CAD build for the part. Positions are in the model's coordinates, mm. A direction names the side the tool comes from. Round coordinates to 2 decimals unless told otherwise and drop trailing zeros. Loops run counter-clockwise (first coordinate to the right, second up) from the corner with the lowest first, then second, coordinate; pieces in that order, holes last. Notation, with made-up numbers: (53, 8.5) - (67, 8.5) arc R30 cw to (67, 37.5) - close; hole circle Ø5 at (8, 80.5). An arc over 180 degrees is marked (long way). Use one line per item in the form item = value.
from build123d import *

# Parameters (mm, degrees)
SKETCH1_R                    = 2.475
BOSS_EXTRUDE1_DEPTH          = 30.2
SKETCH2_R                    = 5
BOSS_EXTRUDE2_DEPTH          = 3
M2_5X0_45_TAPPED_HOLE2_D     = 2.05
M2_5X0_45_TAPPED_HOLE2_DEPTH = 7.25
M2_5X0_45_TAPPED_HOLE2_TIP   = 0.615882135
CUT_EXTRUDE1_DEPTH           = 1


with BuildPart() as part:
    # Sketch1 → Boss-Extrude1 (new body)
    with BuildSketch(Plane(origin=(0, 0, 0), x_dir=(1, 0, 0), z_dir=(0, 1, 0))):
        with Locations(Location((0, 0, 0), (0, 0, 270))):
            Circle(SKETCH1_R)
    extrude(amount=BOSS_EXTRUDE1_DEPTH)

    # Sketch2 → Boss-Extrude2 (add)
    with BuildSketch(Plane(origin=(0, 30.2, 0), x_dir=(1, 0, 0), z_dir=(0, 1, 0))):
        with Locations(Location((0, 0, 0), (0, 0, 270))):
            Circle(SKETCH2_R)
    extrude(amount=BOSS_EXTRUDE2_DEPTH)

    # M2.5x0.45 Tapped Hole2
    with Locations(Plane(origin=(0, 0, 0), x_dir=(-1, 0, 0), z_dir=(0, -1, 0))):
        with Locations((0, 0)):
            Hole(M2_5X0_45_TAPPED_HOLE2_D / 2, depth=M2_5X0_45_TAPPED_HOLE2_DEPTH)
            with Locations((0, 0, -(M2_5X0_45_TAPPED_HOLE2_DEPTH + M2_5X0_45_TAPPED_HOLE2_TIP / 2))):  # 118° drill point
                Cone(0, M2_5X0_45_TAPPED_HOLE2_D / 2, M2_5X0_45_TAPPED_HOLE2_TIP, mode=Mode.SUBTRACT)

    # Sketch15 → Cut-Extrude1 (cut)
    with BuildSketch(Plane(origin=(0, 33.2, 0), x_dir=(1, 0, 0), z_dir=(0, 1, 0))):
        with BuildLine():
            Line((-1.233974359, 1.812951114), (-0.36318109, 1.812951114))
            add(Edge.make_bspline(
                [(-0.36318109, 1.812951114), (-0.320639792, 1.81277482), (-0.238097313, 1.812432758), (-0.117944897, 1.807143974), (-0.005417149, 1.799981229), (0.099544539, 1.788516219), (0.196648731, 1.774795951), (0.286334292, 1.758075463), (0.368386787, 1.738061375), (0.466181104, 1.706551189), (0.577385314, 1.659544464), (0.69854813, 1.590428983), (0.803039094, 1.505102662), (0.877878706, 1.423867273), (0.929466312, 1.354120247), (0.962333975, 1.29956986), (0.991258246, 1.244562421), (1.014994605, 1.187686093), (1.03202411, 1.128998157), (1.044819465, 1.069026747), (1.052748306, 1.007805904), (1.053904509, 0.96648646), (1.054487179, 0.945663454)],
                knots=[0, 0, 0, 0, 1.369395837, 2.657025819, 3.871165245, 4.998641136, 6.055205263, 7.027626947, 7.93453697, 8.772070297, 10.33297941, 11.813084282, 13.246620381, 14.657649904, 15.357394331, 16.036113692, 16.705765142, 17.356858567, 18.01624541, 18.669941831, 19.32971487, 20, 20, 20, 20], degree=3))
            add(Edge.make_bspline(
                [(1.054487179, 0.945663454), (1.052654691, 0.906966077), (1.049036329, 0.83055573), (1.022472193, 0.718394704), (0.976599056, 0.612617091), (0.914657599, 0.512329552), (0.835047458, 0.419836309), (0.738822803, 0.335989818), (0.625254813, 0.261839362), (0.541323489, 0.221824121), (0.497796474, 0.201072108)],
                knots=[0, 0, 0, 0, 0.940699359, 1.857468692, 2.784365282, 3.733848908, 4.713424377, 5.740520916, 6.828227955, 8, 8, 8, 8], degree=3))
            add(Edge.make_bspline(
                [(0.497796474, 0.201072108), (0.551768458, 0.185885857), (0.654151048, 0.157078178), (0.796065663, 0.105389985), (0.918408451, 0.049772841), (1.022231895, -0.011295733), (1.110522963, -0.078039162), (1.189022557, -0.14879913), (1.255397333, -0.227838547), (1.312111012, -0.312229672), (1.356926733, -0.401765633), (1.389714175, -0.495676987), (1.410030166, -0.593359641), (1.412313767, -0.660043172), (1.413461538, -0.693559303)],
                knots=[0, 0, 0, 0, 1.455388961, 2.760811819, 3.917406684, 4.940403342, 5.880962759, 6.78714742, 7.678335857, 8.55349333, 9.421892728, 10.270128957, 11.13054119, 12, 12, 12, 12], degree=3))
            add(Edge.make_bspline(
                [(1.413461538, -0.693559303), (1.412242032, -0.727766419), (1.409835393, -0.795272532), (1.390894564, -0.894196499), (1.36088474, -0.989122853), (1.317295116, -1.079552584), (1.262055501, -1.166202634), (1.195329189, -1.249512571), (1.114856404, -1.327158434), (1.024464106, -1.401484855), (0.922871793, -1.468011987), (0.813113979, -1.527831578), (0.693968983, -1.576136638), (0.567314142, -1.617190861), (0.43218615, -1.648584594), (0.288953701, -1.670407593), (0.137495898, -1.685226372), (0.033691266, -1.686430398), (-0.01963141, -1.687048886)],
                knots=[0, 0, 0, 0, 0.84636283, 1.670256716, 2.484525081, 3.304937408, 4.147653302, 5.024173689, 5.940669469, 6.911204725, 7.917390592, 8.942545822, 10.000945251, 11.095161556, 12.236182265, 13.430964445, 14.680330095, 16, 16, 16, 16], degree=3))
            Line((-0.01963141, -1.687048886), (-1.233974359, -1.687048886))
            Line((-1.233974359, -1.687048886), (-1.233974359, 1.812951114))
        make_face()
        with BuildLine():
            Line((-0.78525641, 1.453976755), (-0.78525641, 0.332181883))
            Line((-0.78525641, 0.332181883), (-0.534254808, 0.332181883))
            add(Edge.make_bspline(
                [(-0.534254808, 0.332181883), (-0.497329505, 0.332581376), (-0.426039685, 0.333352655), (-0.322906469, 0.335567073), (-0.227348255, 0.341740614), (-0.139336138, 0.348009662), (-0.058900721, 0.357993139), (0.013762316, 0.370008339), (0.079332379, 0.382624131), (0.154899034, 0.404259896), (0.240417473, 0.435647338), (0.332105819, 0.484931753), (0.412678402, 0.543856716), (0.481314845, 0.611394969), (0.536663448, 0.686573824), (0.57599864, 0.767139114), (0.601758026, 0.851788302), (0.604422567, 0.909955529), (0.605769231, 0.939353358)],
                knots=[0, 0, 0, 0, 1.228781612, 2.372346689, 3.431775579, 4.414692591, 5.307870858, 6.127357932, 6.865508947, 7.527788984, 8.741043829, 9.889226724, 10.97954299, 12.051822853, 13.081523397, 14.06922767, 15.024183967, 16, 16, 16, 16], degree=3))
            add(Edge.make_bspline(
                [(0.605769231, 0.939353358), (0.605069578, 0.958793616), (0.603694839, 0.996991554), (0.593661455, 1.052580133), (0.577534344, 1.105242414), (0.554328035, 1.154703777), (0.5237272, 1.200237525), (0.487498602, 1.243054995), (0.444430933, 1.282429509), (0.394180863, 1.318194021), (0.336986398, 1.350636833), (0.272169726, 1.378747532), (0.199333131, 1.401261658), (0.119403459, 1.421298849), (0.031136116, 1.435282122), (-0.064476809, 1.446778275), (-0.168191884, 1.452820409), (-0.239777112, 1.453581571), (-0.276943109, 1.453976755)],
                knots=[0, 0, 0, 0, 0.81361945, 1.598671385, 2.356922644, 3.11416307, 3.876758201, 4.647284559, 5.457543271, 6.312925357, 7.224393372, 8.206010094, 9.264318981, 10.412951858, 11.653205513, 13.002848701, 14.443923124, 16, 16, 16, 16], degree=3))
            Line((-0.276943109, 1.453976755), (-0.78525641, 1.453976755))
        make_face(mode=Mode.SUBTRACT)
        with BuildLine():
            Line((-0.78525641, -0.026792476), (-0.78525641, -1.328074527))
            Line((-0.78525641, -1.328074527), (-0.239783654, -1.328074527))
            add(Edge.make_bspline(
                [(-0.239783654, -1.328074527), (-0.200987304, -1.327690356), (-0.125956017, -1.326947378), (-0.017469258, -1.324522225), (0.083100767, -1.3191041), (0.17537521, -1.31032603), (0.259927106, -1.301113071), (0.336165219, -1.288439684), (0.40454898, -1.273893981), (0.483978905, -1.251863739), (0.573325451, -1.217636717), (0.669712619, -1.165152633), (0.75566181, -1.103329109), (0.828970911, -1.03131561), (0.888686141, -0.952756222), (0.932418672, -0.869523141), (0.96005753, -0.782699587), (0.963185334, -0.723201137), (0.96474359, -0.693559303)],
                knots=[0, 0, 0, 0, 1.229962997, 2.378721407, 3.439847587, 4.421852365, 5.31694785, 6.13545284, 6.87076298, 7.532272478, 8.747192924, 9.894301625, 11.002789606, 12.092524487, 13.140140875, 14.117719788, 15.062257293, 16, 16, 16, 16], degree=3))
            add(Edge.make_bspline(
                [(0.96474359, -0.693559303), (0.964248878, -0.675063946), (0.963265781, -0.638309743), (0.954024974, -0.584078298), (0.937930082, -0.532037628), (0.91842641, -0.48095885), (0.889767871, -0.433133136), (0.857272369, -0.385843714), (0.817562099, -0.341127783), (0.772510175, -0.298244001), (0.722331889, -0.257897223), (0.667454581, -0.22063784), (0.608022441, -0.186922123), (0.544201506, -0.155945118), (0.47544777, -0.128829439), (0.402387834, -0.105003984), (0.324849413, -0.084628111), (0.271392504, -0.073739953), (0.243990385, -0.068158662)],
                knots=[0, 0, 0, 0, 0.855972342, 1.700998913, 2.536409134, 3.376362511, 4.224639329, 5.110263021, 6.030513101, 6.987259223, 7.987740375, 9.008211689, 10.055134299, 11.148935388, 12.290305944, 13.47432859, 14.705335734, 16, 16, 16, 16], degree=3))
            add(Edge.make_bspline(
                [(0.243990385, -0.068158662), (0.223684811, -0.064699565), (0.179484109, -0.057169883), (0.107606648, -0.049320661), (0.025555986, -0.042263275), (-0.066812959, -0.037035463), (-0.169619858, -0.031670757), (-0.283016111, -0.029566976), (-0.406639983, -0.027064663), (-0.492419411, -0.02688564), (-0.537059295, -0.026792476)],
                knots=[0, 0, 0, 0, 0.631265822, 1.374124787, 2.215341576, 3.155543556, 4.209810819, 5.370695037, 6.631701453, 8, 8, 8, 8], degree=3))
            Line((-0.537059295, -0.026792476), (-0.78525641, -0.026792476))
        make_face(mode=Mode.SUBTRACT)
    extrude(amount=-CUT_EXTRUDE1_DEPTH, mode=Mode.SUBTRACT)


solid = part.part
1) Drill centre lines: probe 1 along Y at (x, z) = (4.5, 1.25); probe 2 along Y at (x, z) = (-0.25, -1.5); probe 3 along Z at (x, y) = (0.25, 30). Where is each one in solid material? Low to high.
Report:
probe_1 = 30.2 to 33.2
probe_2 = 0 to 32.2
probe_3 = -2.46 to 2.46
2) Slice it at B-B (y = 5). Write the cut outline in (x, z) (3 decimals).
Report:
outline = circle Ø4.95 at (0, 0); hole circle Ø2.05 at (0, 0)
3) Slice it at A-A (z = 2). Write the cut outline in (x, y), plus the area to 3 significant figures.
Report:
outline = (-4.58, 30.2) - (-1.46, 30.2) - (-1.46, 0) - (1.46, 0) - (1.46, 30.2) - (4.58, 30.2) - (4.58, 33.2) - (-4.58, 33.2) - close
area = 116 mm^2
4) Tool access for faces 1 (the flat face through (1.2, 33.2, -0.1)), 2 (the flat face through (-0.785, 33, 1)), 3 (the cylindrical face through (0.74, 14.89, 2.36)): list every direction of +Z, -Z, +X, -X, +Y, -Y with a clear straight run to the whole face (end or side of a thin tool).
Report:
face_1 = +Z, -Z, +X, -X, +Y
face_2 = +Y
face_3 = -Y
5) Flat gauge pins, fed straight in: pin 1 (5 mm diameter, centred on y = 12.5, z = -2.5, fed in from -X) (3 decimals); pin 2 (0.6 mm diameter, centred on x = -0.5, y = 33, fed in from -Z); pin 3 (4 mm diameter, centred on x = -1, y = 28, fed in from +Z) (3 decimals). Where does each tip first touch, or does it go through?
Report:
pin_1 = -2.475
pin_2 = -5
pin_3 = 2.475
6) Slice it at C-C (y = 28). Write the cut outline in (x, z) (3 decimals), plus the area to 3 significant figures.
Report:
outline = circle Ø4.95 at (0, 0)
area = 19.2 mm^2
7) Slice it at D-D (x = -3.75). Write the cut outline in (y, z).
Report:
outline = (30.2, -3.31) - (33.2, -3.31) - (33.2, 3.31) - (30.2, 3.31) - close
8) Two-plate mould, pull along X, no slides. Class faces 4 (the flat face through (-1, 33, -1.813)), 5 (the cylindrical face through (-4.88, 31.68, -1.08)), 6 (the flat face through (0, 33.2, 1)): +X half, -X half, draft (parallel to the pull), parting line (faces both ways), or undercut.
Report:
face_4 = undercut
face_5 = parting line
face_6 = draft
